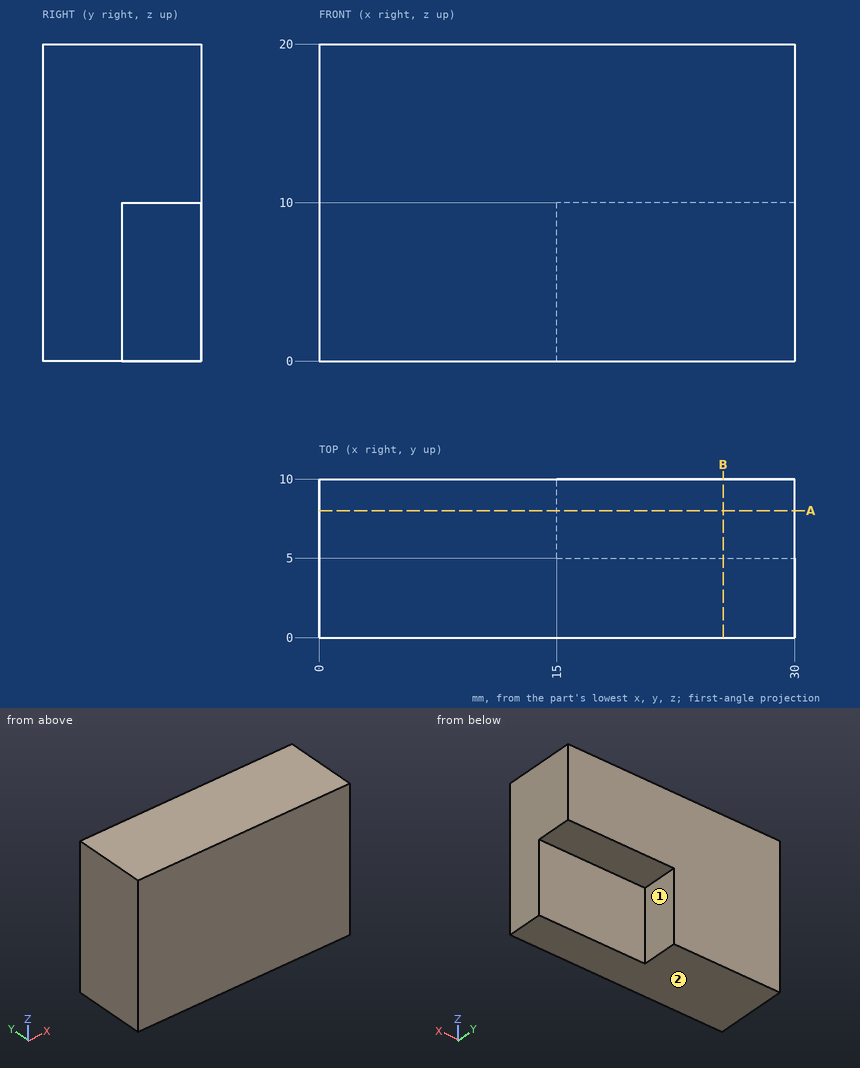
Can you work these out from the drawing? Everything is in mm from the part's minimum corner. A direction names the side the tool comes from. Give positions to 0.01 mm unless a question says otherwise; leave off trailing zeros. Loops run counter-clockwise (first coordinate to the right, second up) from the corner with the lowest first, then second, coordinate; pieces in that order, holes last. Notation, with made-up numbers: (6.25, 10) -> (14.25, 10) arc R14 cw to (14.25, 37) -> close; hole circle Ø1 at (23, 3.25). An arc over 180 degrees is marked (long way). Return JSON: item names as keys, results as strings.
Q1. On a 3-axis mill with a long thin cutter (end or side, diameter ignored), from which of +Z, -Z, +X, -X, +Y, -Y can I reach the whole of each face in a straight line? I mean the marked faces 1 and 2. Say none if no direction works.
Checks:
{"face 1": "-Z, +X, +Y", "face 2": "-Z, +X, -X, +Y, -Y"}
Q2. For pin 1 Ø3 at (x, z) = (24, 5.5) entering from +Y; pin 2 Ø5.5 at (y, z) = (8, 7) entering from +X; pin 3 Ø4 at (y, z) = (9, 15) entering from -X; pin 4 Ø2.5 at (x, y) = (19.5, 8.5) entering from -Z, each with a flat end and sliding along its axis, tell me the tip position at first contact or that it passes through.
Checks:
{"pin 1": "stops at y = 5", "pin 2": "stops at x = 15", "pin 3": "stops at x = 0", "pin 4": "stops at z = 10"}
Q3. I want a section at B-B, the plane x = 25.5. List the corners of the cut face in (y, z) for me.
Checks:
{"outline": "(0, 0) -> (5, 0) -> (5, 10) -> (10, 10) -> (10, 20) -> (0, 20) -> close"}
Q4. I want a section at A-A, the plane y = 8. List the corners of the cut face in (x, z) for me.
Checks:
{"outline": "(0, 0) -> (15, 0) -> (15, 10) -> (30, 10) -> (30, 20) -> (0, 20) -> close"}
Q5. I need wall thicknesses on probe 1 along Z at (x, y) = (28.75, 5.5); probe 2 along X at (y, z) = (8.75, 2.75); probe 3 along Y at (x, z) = (18.25, 1.5). Which ranges of each line are inside material? Lowest first, please.
Checks:
{"probe 1": "z = 10 to 20", "probe 2": "x = 0 to 15", "probe 3": "y = 0 to 5"}
